Geometry check sheet. Reference: the model listing, model coordinates, mm. A direction names the side the tool comes from. Coordinates: 2 decimals unless noted, no trailing zeros. Write each loop counter-clockwise with the first axis right and the second up, starting at its lowest first coordinate (ties: lowest second). Pieces come first, ordered by that corner, then holes.
Solid Edge part; units mm, degrees
sketch "Sketch1" plane through (0, 0, 0) normal (0, -1, 0) x (1, 0, 0)
  circle A0 centre (0, 0) radius 1.5
extrude "Protrusion1" add sketch "Sketch1" against normal blind 6
sketch "Sketch2" plane through (0, 6, 0) normal (0, 1, 0) x (0, 0, -1)
  circle A0 centre (0, 0) radius 2.5
extrude "ExtrudedProtrusion_2" add sketch "Sketch2" along normal blind 8
sketch "Sketch3" plane through (0, 14, 0) normal (0, 1, 0) x (-1, 0, 0)
  circle A0 centre (0, 0) radius 1.05
extrude "ExtrudedCutout_1" cut sketch "Sketch3" against normal blind 5
1. Sectioned sample at D-D, the plane y = 1. Record the boundary of the cut face in (x, z), and give its area (3 significant figures).
Computed values:
outline: circle Ø3 at (0, 0)
area: 7.07 mm2
2. Access from +Z, -Z, +X, -X, +Y, -Y to the whole of each face (thin tool, end or side, straight path). Record for faces 1 (the cylindrical face through (-1, 11.54, 0.32)), 2 (the flat face through (-1, 14, 1)), 3 (the flat face through (0, 6, 2)).
Computed values:
face 1: +Y
face 2: +Z, -Z, +X, -X, +Y
face 3: -Y
3. Sectioned sample at C-C, the plane y = 10. Record the boundary of the cut face in (x, z), and give its area (3 significant figures).
Computed values:
outline: circle Ø5 at (0, 0); hole circle Ø2.1 at (0, 0)
area: 16.2 mm2
4. Draft check along X on faces 4 (the cylindrical face through (-2.44, 9.94, 0.54)), 5 (the flat face through (0, 9, 0)), 6 (the flat face through (0, 0, 0)). Enter one of: released by +X, released by -X, zero draft, split by the parting line, or undercut.
Computed values:
face 4: split by the parting line
face 5: undercut
face 6: zero draft
5. Sectioned sample at B-B, the plane z = 0. Record the boundary of the cut face in (x, y).
Computed values:
outline: (-2.5, 6) - (-1.5, 6) - (-1.5, 0) - (1.5, 0) - (1.5, 6) - (2.5, 6) - (2.5, 14) - (1.05, 14) - (1.05, 9) - (-1.05, 9) - (-1.05, 14) - (-2.5, 14) - close
6. Gauge pin test, flat ends, axial feed: pin 1 Ø2 at (x, y) = (0, 2.5) entering from +Z; pin 2 Ø0.6 at (x, z) = (0, -0.5) entering from +Y; pin 3 Ø1 at (x, y) = (1, 2.5) entering from -Z. Record the tip position at first contact, or that the pin passes through.
Computed values:
pin 1: stops at z = 1.5
pin 2: stops at y = 9
pin 3: stops at z = -1.41
7. Sectioned sample at A-A, the plane x = 0. Record the boundary of the cut face in (y, z).
Computed values:
outline: (0, -1.5) - (6, -1.5) - (6, -2.5) - (14, -2.5) - (14, -1.05) - (9, -1.05) - (9, 1.05) - (14, 1.05) - (14, 2.5) - (6, 2.5) - (6, 1.5) - (0, 1.5) - close
8. Thickness scan on line 1 along Z through (x, y) = (0, 11.85); line 2 along Y through (x, z) = (1.85, 1.55); line 3 along Y through (x, z) = (-0.45, 0.2). Record the ranges inside material, lowest first.
Computed values:
line 1: z = -2.5 to -1.05, 1.05 to 2.5
line 2: y = 6 to 14
line 3: y = 0 to 9
